from build123d import *

# Parameters (mm, degrees)
BOSS_EXTRUDE1_DEPTH = 8
SKETCH3_R           = 1.6
CUT_EXTRUDE1_DEPTH  = 10
SKETCH4_R           = 2
CUT_EXTRUDE2_DEPTH  = 10


with BuildPart() as part:
    # Sketch1 → Boss-Extrude1 (new body)
    with BuildSketch(Plane(origin=(0, 0, 0), x_dir=(0, 0, -1), z_dir=(1, 0, 0))):
        Polygon((70.223325062, 25.017667028), (82.223325062, 25.017667028), (82.223325062, 31.017667028), (84.223325062, 31.017667028), (84.223325062, 21.017667028), (74.223325062, 21.017667028), (74.223325062, -2), (70.223325062, -2), (60.223325062, -2), (60.223325062, 0), (67.723325062, 0), (70.223325062, 2.5), align=None)
    extrude(amount=BOSS_EXTRUDE1_DEPTH)

    # Sketch3 → Cut-Extrude1 (cut)
    with BuildSketch(Plane.XY.offset(-82.223325062)):
        with Locations((4, 28.017667028)):
            Circle(SKETCH3_R)
    extrude(amount=-CUT_EXTRUDE1_DEPTH, mode=Mode.SUBTRACT)

    # Sketch4 → Cut-Extrude2 (cut)
    with BuildSketch(Plane(origin=(0, 0, 0), x_dir=(1, 0, 0), z_dir=(0, 1, 0))):
        with Locations(Location((4, 65.223325062, 0), (0, 0, 270))):
            Circle(SKETCH4_R)
    extrude(amount=-CUT_EXTRUDE2_DEPTH, mode=Mode.SUBTRACT)


solid = part.part
Can you work these out from the model? Positions are in its coordinate system, mm. A direction names the side the tool comes from. Give positions to 0.01 mm unless a question says otherwise; leave off trailing zeros. Loops run counter-clockwise (first coordinate to the right, second up) from the corner with the lowest first, then second, coordinate; pieces in that order, holes last. Notation, with made-up numbers: M 30.5,88.25 L 84.5,88.25 A9 cw 84.5,97.25 Z; hole C 50.25,55.25 d1. An arc over 180 degrees is marked long. One line per item, written item: value.
1) Imagine slicing it at D-D on y = 20. Write out the boundary of the cut face in (x, z).
Geometry check:
outline: M 0,-74.22 L 8,-74.22 L 8,-70.22 L 0,-70.22 Z
2) Thinking about a two-plate mould opening in Z: for faces 1 (the face through (4.09, -0.99, -67.22)), 2 (the face through (4, 26, -84.223)), 3 (the face through (4, 14, -70.223)), 4 (the face through (4, 21.018, -79)), which applies, +Z half, -Z half, draft (parallel to the pull), parting line (faces both ways), or undercut?
Geometry check:
face 1: undercut
face 2: -Z half
face 3: +Z half
face 4: draft
3) I'm going to push flat-ended pins straight in: pin 1 (4 mm diameter, centred on x = 2.5, z = -77, fed in from -Y); pin 2 (1.9 mm diameter, centred on x = 4, y = 28.02, fed in from -Z); pin 3 (8 mm diameter, centred on y = 9, z = -68, fed in from -X); pin 4 (4 mm diameter, centred on x = 1, z = -66, fed in from +Y). Where does each tip first touch, or does it pass through?
Geometry check:
pin 1: stops at y = 21.02
pin 2: passes through
pin 3: stops at x = 0
pin 4: stops at y = 0.28
4) Imagine slicing it at B-B on y = 28.5. Write out the boundary of the cut face in (x, z), and give its area (3 significant figures).
Geometry check:
outline: M 0,-84.22 L 2.47,-84.22 L 2.47,-82.22 L 0,-82.22 Z; M 5.53,-84.22 L 8,-84.22 L 8,-82.22 L 5.53,-82.22 Z
area: 9.90 mm²
5) Imagine slicing it at C-C on x = 1. Write out the boundary of the cut face in (y, z), and give its area (3 significant figures).
Geometry check:
outline: M -2,-74.22 L 21.02,-74.22 L 21.02,-84.22 L 31.02,-84.22 L 31.02,-82.22 L 25.02,-82.22 L 25.02,-70.22 L 2.5,-70.22 L 0,-67.72 L 0,-60.22 L -2,-60.22 Z
area: 183 mm²
6) Imagine slicing it at A-A on x = 4. Write out the boundary of the cut face in (y, z), and give its area (3 significant figures).
Geometry check:
outline: M -2,-74.22 L 21.02,-74.22 L 21.02,-84.22 L 26.42,-84.22 L 26.42,-82.22 L 25.02,-82.22 L 25.02,-70.22 L 2.5,-70.22 L 0,-67.72 L 0,-67.22 L -2,-67.22 Z; M -2,-63.22 L 0,-63.22 L 0,-60.22 L -2,-60.22 Z; M 29.62,-84.22 L 31.02,-84.22 L 31.02,-82.22 L 29.62,-82.22 Z
area: 169 mm²
7) Please list where these lines run through material, in increasing order: line 1 (Y direction, x = 4, z = -83.45); line 2 (Y direction, x = 6.25, z = -78.25); line 3 (Y direction, x = 7, z = -67).
Geometry check:
line 1: y = 21.02 to 26.42, 29.62 to 31.02
line 2: y = 21.02 to 25.02
line 3: y = -2 to 0
8) On a 3-axis mill with a long thin cutter (end or side, diameter ignored), from which of +Z, -Z, +X, -X, +Y, -Y can I reach the whole of each face in a straight line? I mean faces 5 (the face through (2, 28, -82.223)), 6 (the face through (4, 31.018, -83)), 7 (the face through (4, 10, -74.223)). Say none if no direction works.
Geometry check:
face 5: +Z, +X, -X, +Y
face 6: +Z, -Z, +X, -X, +Y
face 7: -Z, +X, -X, -Y
